```python
from build123d import *
from build123d.topology import SkipClean

# Parameters (mm, degrees)
SKETCH1_W                            = 4.75
SKETCH1_H                            = 7
FILLET1_R                            = 1
SKETCH16_W                           = 16
SKETCH16_H                           = 1
CUT_EXTRUDE5_DEPTH                   = 1
CUT_EXTRUDE5_DIRECTION_2_REACH       = 18.492
CUT_EXTRUDE6_REACH                   = 15.304
SKETCH17_W                           = 3.5
SKETCH17_H                           = 5.261387212
CUT_EXTRUDE7_DEPTH                   = 18.408690359
CUT_EXTRUDE7_DEPTH_BACK              = 18.408690359
SKETCH18_R                           = 1.2
CUT_EXTRUDE10_START                  = -6
SKETCH21_R                           = 1.6
CUT_EXTRUDE10_DEPTH                  = 6
CUT_EXTRUDE11_DEPTH                  = 18.26991621
CUT_EXTRUDE11_DEPTH_BACK             = 18.26991621
SKETCH22_R                           = 1.2
CUT_EXTRUDE9_REACH                   = 20.603
CUT_EXTRUDE9_END_RADIUS              = 8
SKETCH20_R                           = 1.2
CUT_EXTRUDE12_REACH                  = 21.585
SKETCH19_R                           = 2.25
CUT_EXTRUDE13_REACH                  = 21.585
CUT_EXTRUDE13_END_RADIUS             = 8
SKETCH24_R                           = 2.25
CUT_EXTRUDE14_REACH                  = 18.492
CUT_EXTRUDE14_END_RADIUS             = 8
SKETCH25_W                           = 2.25
SKETCH25_H                           = 1
CUT_EXTRUDE14_DIRECTION_2_REACH      = 18.492
CUT_EXTRUDE14_DIRECTION_2_END_RADIUS = 8
M2_5_CLEARANCE_HOLE1_D               = 2.9
M2_5_CLEARANCE_HOLE1_DEPTH           = 8.029752102
M2_5_CLEARANCE_HOLE1_TIP             = 0.871247898
CUT_EXTRUDE15_START                  = -12
SKETCH29_W                           = 4
SKETCH29_H                           = 2.25
CUT_EXTRUDE15_DEPTH                  = 12
FILLET3_R                            = 0.25
SKETCH30_R                           = 8
CUT_EXTRUDE19_DEPTH                  = 1
BOSS_EXTRUDE1_START                  = 1
BOSS_EXTRUDE1_DEPTH                  = 1


with BuildPart() as part:
    # Sketch1 → Revolve1 (revolve)
    with BuildSketch(Plane.XY, mode=Mode.PRIVATE) as revolve1_sk:
        with Locations((5.625, 3.5)):
            Rectangle(SKETCH1_W, SKETCH1_H)
    revolve(revolve1_sk.sketch.rotate(Axis((0, 0, 0), (0, 1, 0)), 90), axis=Axis((0, 0, 0), (0, 1, 0)))

    # Sketch1<3> → Revolve2 (revolve)
    with BuildSketch(Plane.XY, mode=Mode.PRIVATE) as revolve2_sk:
        Polygon((1.6, 7), (3.25, 7), (8, 7), (8, 12), (1.6, 12), align=None)
    revolve(revolve2_sk.sketch.rotate(Axis((0, 0, 0), (0, 1, 0)), 90), axis=Axis((0, 0, 0), (0, 1, 0)))

    # Fillet1
    fillet1_edges = [part.edges().sort_by_distance(p)[0] for p in [
        (0, 12, 8),
    ]]
    fillet(fillet1_edges, radius=FILLET1_R)

    # Sketch16 → Cut-Extrude5 (cut)
    with BuildSketch(Plane.XY):
        with Locations((0, 5.5)):
            Rectangle(SKETCH16_W, SKETCH16_H)
    extrude(amount=-CUT_EXTRUDE5_DEPTH, mode=Mode.SUBTRACT)

    # Sketch16 → Cut-Extrude5 direction 2 (cut, up to next)
    with BuildSketch(Plane.XY, mode=Mode.PRIVATE) as cut_extrude5_direction_2_sk1:
        with Locations((0, 5.5)):
            Rectangle(SKETCH16_W, SKETCH16_H)
    cut_extrude5_direction_2_tool1 = extrude(cut_extrude5_direction_2_sk1.sketch, amount=CUT_EXTRUDE5_DIRECTION_2_REACH, mode=Mode.PRIVATE) & part.part
    add(cut_extrude5_direction_2_tool1.solids().sort_by_distance((0, 5.5, 0))[0], mode=Mode.SUBTRACT)

    # Sketch17 → Cut-Extrude6 (cut, up to next)
    with BuildSketch(Plane(origin=(0, 5, 0), x_dir=(1, 0, 0), z_dir=(0, 1, 0)), mode=Mode.PRIVATE) as cut_extrude6_sk1:
        with Locations((0, -5.369306394)):
            Rectangle(SKETCH17_W, SKETCH17_H)
    cut_extrude6_tool1 = extrude(cut_extrude6_sk1.sketch, amount=-CUT_EXTRUDE6_REACH, mode=Mode.PRIVATE) & part.part
    add(cut_extrude6_tool1.solids().sort_by_distance((0, 5, 5.369306))[0], mode=Mode.SUBTRACT)

    # Sketch18 → Cut-Extrude7 (cut, two sides: drawn at the far end of the back side and taken through both)
    with BuildSketch(Plane.ZY.offset(-1.75).offset(-CUT_EXTRUDE7_DEPTH_BACK)):
        with Locations((4.772430143, 2.5)):
            Circle(SKETCH18_R)
    extrude(amount=CUT_EXTRUDE7_DEPTH + CUT_EXTRUDE7_DEPTH_BACK, mode=Mode.SUBTRACT)

    # Sketch21 → Cut-Extrude10 (cut)
    with BuildSketch(Plane(origin=(0, 12, 0), x_dir=(1, 0, 0), z_dir=(0, 1, 0)).offset(CUT_EXTRUDE10_START)):
        Circle(SKETCH21_R)
        Polygon((-1.5, -1.9), (-1.5, -11.891029443), (1.5, -11.891029443), (1.5, -1.9), (1.322875656, -1.9), (1.322875656, -0.9), (-1.322875656, -0.9), (-1.322875656, -1.9), align=None)
    extrude(amount=CUT_EXTRUDE10_DEPTH, mode=Mode.SUBTRACT)

    # Sketch22 → Cut-Extrude11 (cut, two sides: drawn at the far end of the back side and taken through both)
    with BuildSketch(Plane(origin=(-1.5, 0, 0), x_dir=(0, 0, -1), z_dir=(1, 0, 0)).offset(-CUT_EXTRUDE11_DEPTH_BACK)):
        with Locations((-3.358116823, 8.5)):
            Circle(SKETCH22_R)
    extrude(amount=CUT_EXTRUDE11_DEPTH + CUT_EXTRUDE11_DEPTH_BACK, mode=Mode.SUBTRACT)

    # Cut-Extrude9: up to this cylinder (the profile starts inside it)
    cut_extrude9_end = Plane(origin=(0, 5.9847245, 0), z_dir=(0, -1, 0)) * Cylinder(CUT_EXTRUDE9_END_RADIUS, 65.175449, mode=Mode.PRIVATE)
    # Sketch20 → Cut-Extrude9 (cut, up to the surface)
    with BuildSketch(Plane(origin=(-3.75, 0, 0), x_dir=(0, 0, -1), z_dir=(1, 0, 0)), mode=Mode.PRIVATE) as cut_extrude9_sk1:
        Polygon((-2.463029066, 2.5), (-3.617729604, 4.5), (-5.927130681, 4.5), (-7.08183122, 2.5), (-5.927130681, 0.5), (-3.617729604, 0.5), align=None)
    cut_extrude9_tool1 = extrude(cut_extrude9_sk1.sketch, amount=-CUT_EXTRUDE9_REACH, mode=Mode.PRIVATE) & cut_extrude9_end
    add(cut_extrude9_tool1.solids().sort_by_distance((-3.75, 2.5, 4.77243))[0], mode=Mode.SUBTRACT)
    # Sketch20 → Cut-Extrude9 (cut, up to the surface)
    with BuildSketch(Plane(origin=(-3.75, 0, 0), x_dir=(0, 0, -1), z_dir=(1, 0, 0)), mode=Mode.PRIVATE) as cut_extrude9_sk2:
        Polygon((-1.048715746, 8.5), (-2.203416284, 10.5), (-4.512817361, 10.5), (-5.6675179, 8.5), (-4.512817361, 6.5), (-2.203416284, 6.5), align=None)
        with Locations((-3.358116823, 8.5)):
            Circle(SKETCH20_R, mode=Mode.SUBTRACT)
    cut_extrude9_tool2 = extrude(cut_extrude9_sk2.sketch, amount=-CUT_EXTRUDE9_REACH, mode=Mode.PRIVATE) & cut_extrude9_end
    add(cut_extrude9_tool2.solids().sort_by_distance((-3.75, 9.469449, 1.678981))[0], mode=Mode.SUBTRACT)

    # Sketch19 → Cut-Extrude12 (cut, up to next)
    with BuildSketch(Plane.ZY.offset(-5.25), mode=Mode.PRIVATE) as cut_extrude12_sk1:
        with Locations((4.772430143, 2.5)):
            Circle(SKETCH19_R)
    cut_extrude12_tool1 = extrude(cut_extrude12_sk1.sketch, amount=-CUT_EXTRUDE12_REACH, mode=Mode.PRIVATE) & part.part
    add(cut_extrude12_tool1.solids().sort_by_distance((5.25, 2.5, 4.77243))[0], mode=Mode.SUBTRACT)

    # Cut-Extrude13: up to this cylinder (the profile starts inside it)
    cut_extrude13_end = Plane(origin=(0, 8.5, 0), z_dir=(0, -1, 0)) * Cylinder(CUT_EXTRUDE13_END_RADIUS, 60.17, mode=Mode.PRIVATE)
    # Sketch24 → Cut-Extrude13 (cut, up to the surface)
    with BuildSketch(Plane.ZY.offset(-5.25), mode=Mode.PRIVATE) as cut_extrude13_sk1:
        with Locations((3.358116823, 8.5)):
            Circle(SKETCH24_R)
    cut_extrude13_tool1 = extrude(cut_extrude13_sk1.sketch, amount=-CUT_EXTRUDE13_REACH, mode=Mode.PRIVATE) & cut_extrude13_end
    add(cut_extrude13_tool1.solids().sort_by_distance((5.25, 8.5, 3.358117))[0], mode=Mode.SUBTRACT)

    # Cut-Extrude14: up to this cylinder (the profile starts inside it)
    cut_extrude14_end = Plane(origin=(0, 5.5, 0), z_dir=(0, -1, 0)) * Cylinder(CUT_EXTRUDE14_END_RADIUS, 53.984, mode=Mode.PRIVATE)
    # Sketch25 → Cut-Extrude14 (cut, up to the surface)
    with BuildSketch(Plane.ZY, mode=Mode.PRIVATE) as cut_extrude14_sk1:
        with Locations((-2.125, 5.5)):
            Rectangle(SKETCH25_W, SKETCH25_H)
    cut_extrude14_tool1 = extrude(cut_extrude14_sk1.sketch, amount=-CUT_EXTRUDE14_REACH, mode=Mode.PRIVATE) & cut_extrude14_end
    add(cut_extrude14_tool1.solids().sort_by_distance((0, 5.5, -2.125))[0], mode=Mode.SUBTRACT)

    # Cut-Extrude14 direction 2: up to this cylinder (the profile starts inside it)
    cut_extrude14_direction_2_end = Plane(origin=(0, 5.5, 0), z_dir=(0, -1, 0)) * Cylinder(CUT_EXTRUDE14_DIRECTION_2_END_RADIUS, 53.984, mode=Mode.PRIVATE)
    # Sketch25 → Cut-Extrude14 direction 2 (cut, up to the surface)
    with BuildSketch(Plane.ZY, mode=Mode.PRIVATE) as cut_extrude14_direction_2_sk1:
        with Locations((-2.125, 5.5)):
            Rectangle(SKETCH25_W, SKETCH25_H)
    cut_extrude14_direction_2_tool1 = extrude(cut_extrude14_direction_2_sk1.sketch, amount=CUT_EXTRUDE14_DIRECTION_2_REACH, mode=Mode.PRIVATE) & cut_extrude14_direction_2_end
    add(cut_extrude14_direction_2_tool1.solids().sort_by_distance((0, 5.5, -2.125))[0], mode=Mode.SUBTRACT)

    # M2.5 Clearance Hole1
    with Locations(Plane(origin=(0, 0, -8), x_dir=(-1, 0, 0), z_dir=(0, 0, -1))):
        with Locations((0, 8.5), (0, 2.5)):
            Hole(M2_5_CLEARANCE_HOLE1_D / 2, depth=M2_5_CLEARANCE_HOLE1_DEPTH)
            with Locations((0, 0, -(M2_5_CLEARANCE_HOLE1_DEPTH + M2_5_CLEARANCE_HOLE1_TIP / 2))):  # 118° drill point
                Cone(0, M2_5_CLEARANCE_HOLE1_D / 2, M2_5_CLEARANCE_HOLE1_TIP, mode=Mode.SUBTRACT)

    # Sketch29 → Cut-Extrude15 (cut)
    with BuildSketch(Plane(origin=(0, 12, 0), x_dir=(1, 0, 0), z_dir=(0, 1, 0)).offset(CUT_EXTRUDE15_START)):
        with Locations((0, 5.5)):
            Rectangle(SKETCH29_W, SKETCH29_H)
    extrude(amount=CUT_EXTRUDE15_DEPTH, mode=Mode.SUBTRACT)

    # Fillet3
    # the kernel refuses this fillet: 0.25 mm, written as the material it takes off along each edge
    with BuildSketch(Plane(origin=(-1.322875656, 6.402143732, 1.9), x_dir=(-1, 0, 0), z_dir=(0, 1, 0))) as fillet3_piece_1:
        with BuildLine():
            CenterArc((0.25, -0.239142507), FILLET3_R, 106.94793725, 73.05206275)
            Line((0, -0.239142507), (-0.005, -0.239142507))
            Line((-0.005, -0.239142507), (-0.005, 0))
            Line((-0.005, 0), (0, 0.005))
            ThreePointArc((0, 0.005), (0.088562172, 0.005), (0.175666831, 0.00478285))
            Line((0.175666831, 0.00478285), (0.177124344, 0))
        make_face()
    extrude(amount=6.195712537, mode=Mode.SUBTRACT)
    with BuildSketch(Plane(origin=(1.322875656, 6.402143732, 1.9), x_dir=(1, 0, 0), z_dir=(0, 1, 0))) as fillet3_piece_2:
        with BuildLine():
            CenterArc((0.25, 0.239142507), FILLET3_R, 180, 73.05206275)
            Line((0, 0.239142507), (-0.005, 0.239142507))
            Line((-0.005, 0.239142507), (-0.005, 0))
            Line((-0.005, 0), (0, -0.005))
            ThreePointArc((0, -0.005), (0.088562172, -0.005), (0.175666831, -0.00478285))
            Line((0.175666831, -0.00478285), (0.177124344, 0))
        make_face()
    extrude(amount=6.195712537, mode=Mode.SUBTRACT)

    # Sketch30 → Cut-Extrude19 (cut)
    with BuildSketch(Plane(origin=(0, 12, 0), x_dir=(1, 0, 0), z_dir=(0, 1, 0))):
        Circle(SKETCH30_R)
    extrude(amount=-CUT_EXTRUDE19_DEPTH, mode=Mode.SUBTRACT)

    # Sketch31 → Boss-Extrude1 (add)
    with SkipClean():  # the faces are left unmerged after this step: merging them gives an invalid solid
        with BuildSketch(Plane.XZ.offset(-7).offset(BOSS_EXTRUDE1_START)):
            with BuildLine():
                Line((-1.322875656, 0.9), (-1.322875656, 1.660857493))
                ThreePointArc((-1.322875656, 1.660857493), (-1.371979023, 1.809654479), (-1.5, 1.9))
                Line((-1.5, 1.9), (-1.5, 2.883140649))
                ThreePointArc((-1.5, 2.883140649), (0, -3.25), (1.5, 2.883140649))
                Line((1.5, 2.883140649), (1.5, 1.9))
                ThreePointArc((1.5, 1.9), (1.371979023, 1.809654479), (1.322875656, 1.660857493))
                Line((1.322875656, 1.660857493), (1.322875656, 0.9))
                ThreePointArc((1.322875656, 0.9), (0, -1.6), (-1.322875656, 0.9))
            make_face()
        extrude(amount=-BOSS_EXTRUDE1_DEPTH)


solid = part.part
```
Design review of the part built by this model. Coordinates are the model's own, in mm. A direction names the side the tool comes from. Give positions to 0.01 mm unless a question says otherwise; leave off trailing zeros. Write each loop counter-clockwise with the first axis right and the second up, starting at its lowest first coordinate (ties: lowest second). Pieces come first, ordered by that corner, then holes. Notation, with made-up numbers: (53.25, -35) -> (87.25, -35) arc R24 ccw to (87.25, -9) -> close; hole circle Ø4 at (76.25, 44). An arc over 180 degrees is marked (long way). Answer in a Markdown table with one row per item.
(1) Consider section A-A (x = 2.5). State the section outline as (y, z) points.
Results:
| item | result |
|---|---|
| outline | (0, -7.6) -> (11, -7.6) -> (11, 7.6) -> (6, 7.6) -> (6, -3.25) -> (5, -3.25) -> (5, -2.08) -> (0, -2.08) -> close; (0, 2.08) -> (5, 2.08) -> (5, 7.6) -> (0, 7.6) -> close; hole circle Ø2.4 at (2.5, 4.77); hole circle Ø2.4 at (8.5, 3.36) |
(2) Consider section D-D (x = -2.75). State the section outline as (y, z) points, then the cut area to 3 significant figures.
Results:
| item | result |
|---|---|
| outline | (0, -7.51) -> (11, -7.51) -> (11, 7.51) -> (6, 7.51) -> (6, -3.25) -> (5, -3.25) -> (5, -1.73) -> (0, -1.73) -> close; (0, 1.73) -> (5, 1.73) -> (5, 7.51) -> (0, 7.51) -> close; hole circle Ø2.4 at (2.5, 4.77); hole circle Ø2.4 at (8.5, 3.36) |
| area | 128 mm2 |
(3) Consider section C-C (z = -5.5). State the section outline as (x, y) points, then the cut area to 3 significant figures.
Results:
| item | result |
|---|---|
| outline | (-5.81, 0) -> (-2, 0) -> (-2, 11) -> (-5.81, 11) -> close; (2, 0) -> (5.81, 0) -> (5.81, 11) -> (2, 11) -> close |
| area | 83.8 mm2 |
(4) To check wall thickness, follow probe 1 along X at (y, z) = (6.7, 0); probe 2 along X at (y, z) = (1.75, 5.75); probe 3 along Y at (x, z) = (4.5, -2). State the ranges of each line that lie inside material, in increasing order.
Results:
| item | result |
|---|---|
| probe 1 | -8 to -1.6, 1.6 to 8 |
| probe 2 | -3.75 to -1.75, 1.75 to 5.25 |
| probe 3 | 0 to 5, 6 to 11 |
(5) Clearance check with flat-ended pins moving along their axes: pin 1 (2 mm diameter, centred on y = 2.5, z = 4.5, fed in from -X); pin 2 (0.6 mm diameter, centred on y = 9, z = 1.5, fed in from -X); pin 3 (1 mm diameter, centred on x = -4.5, y = 9, fed in from +Z). State where each tip first meets the part, or that it passes through.
Results:
| item | result |
|---|---|
| pin 1 | x = -3.75 |
| pin 2 | x = -7.91 |
| pin 3 | z = 6.93 |
(6) Mouldability with a two-part tool opening along Z and no side actions: class faces 1 (the flat face through (0.1, 5.5, -3.25)), 2 (the flat face through (1.75, 2.5, 6.4)), 3 (the flat face through (-5, 0.5, 5)) as +Z half, -Z half, draft (parallel to the pull), parting line (faces both ways), or undercut.
Results:
| item | result |
|---|---|
| face 1 | +Z half |
| face 2 | draft |
| face 3 | undercut |
(7) Consider section B-B (y = 5.5). State the section outline as (x, z) points (3 decimals).
Results:
| item | result |
|---|---|
| outline | (-7.31, -3.25) arc R8 ccw to (7.31, -3.25) -> close; hole (-2, -6.625) -> (2, -6.625) -> (2, -4.375) -> (-2, -4.375) -> close |
(8) For faces 4 (the flat face through (5.25, 7.5, 4.3)), 5 (the cylindrical face through (1.38, 2.94, -3.79)), 6 (the flat face through (2, 5, -5)), 7 (the flat face through (-6, 10.5, 3)), 8 (the cylindrical face through (-1.659, 2.535, -2.795)), list the 3-axis set-ups (+Z, -Z, +X, -X, +Y, -Y) from which the entire face can be reached by the end or side of a thin tool; tool diameter is ignored.
Results:
| item | result |
|---|---|
| face 4 | +X |
| face 5 | +Z, -Z |
| face 6 | +Y, -Y |
| face 7 | -X |
| face 8 | -Y |
